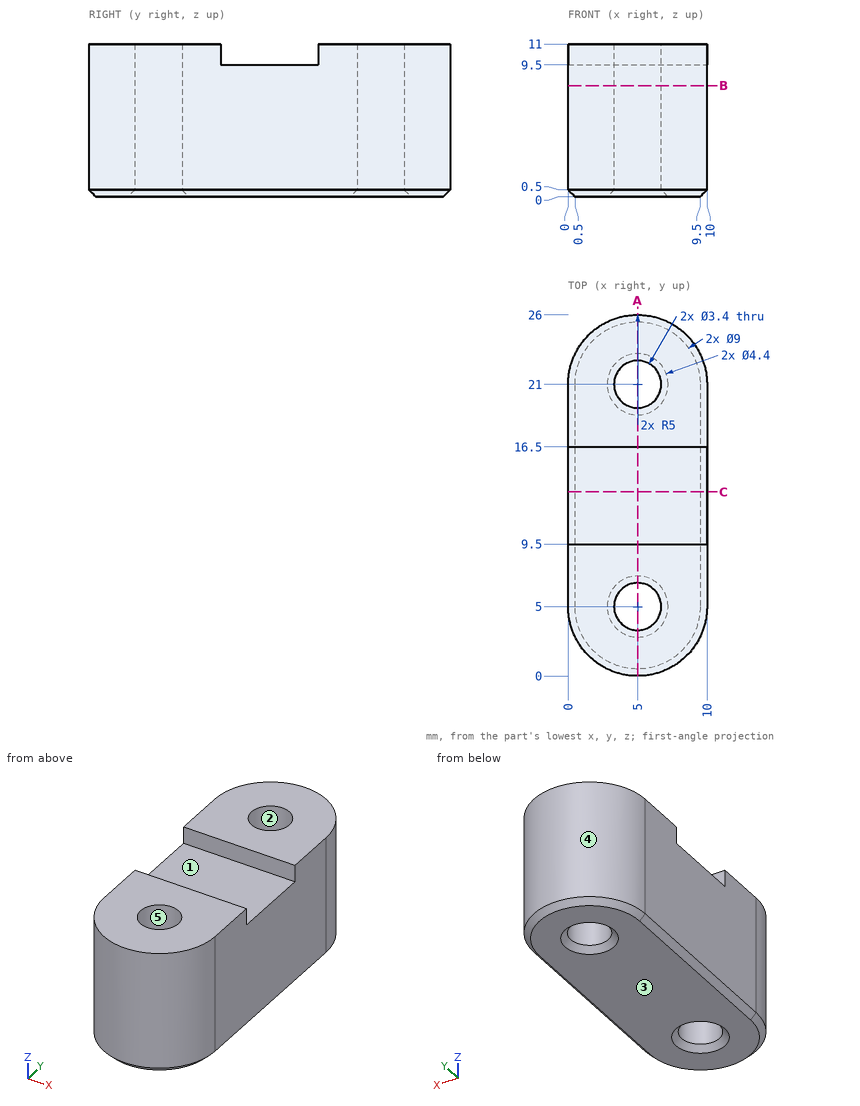
Geometry: see drawing. Coordinates: mm, zero at the bounding-box minimum. A direction names the side the tool comes from. Round coordinates to 2 decimals unless told otherwise and drop trailing zeros. Order: outer loops, then holes, each group sorted by start corner. A loop starts at its lowest first (then second) coordinate and runs counter-clockwise, first axis right, second up. Notation, with made-up numbers: (-15.5, 38) - (23.5, 38) arc R20 cw to (23.5, 56) - close; hole circle Ø10 at (26, 21). An arc over 180 degrees is marked (long way). Use a Markdown table: item, result. Add a question column.
1. First-contact query: pin 1 (0.8 mm diameter, centred on x = 3, z = 10, fed in from -Y); pin 2 (2 mm diameter, centred on x = 3.5, y = 12.5, fed in from +Z); pin 3 (2.5 mm diameter, centred on x = 5, y = 21, fed in from +Z). Flat tips, straight axial feed; report the tip coordinate or a pass-through.
2. Mould query, pull axis X, two halves, no side actions, for the marked faces 3, 4 and 5. Classes: +X half, -X half, draft (parallel to the pull), parting line (faces both ways), or undercut.
3. Section query A-A (x = 5). Return the cut outline in (y, z), then the cut area to 3 significant figures.
4. Set-up query: the marked faces 1 and 2. Return all of +Z, -Z, +X, -X, +Y, -Y with unobstructed straight access to the full face (end or side cutting, diameter ignored); none if empty.
5. Section query C-C (y = 13.25). Return the cut outline in (x, z), then the cut area to 4 significant figures.
6. Section query B-B (z = 8). Return the cut outline in (x, y).
7. Line query: probe 1 along Y at (x, z) = (5, 6.25); probe 2 along Z at (x, y) = (2.75, 12.25); probe 3 along Y at (x, z) = (7.75, 10.75). Output: solid intervals per line, ascending.
Derived:
| question | item | result |
|---|---|---|
| 1 | pin 1 | y = 0.26 |
| 1 | pin 2 | z = 9.5 |
| 1 | pin 3 | through |
| 2 | face 3 | draft |
| 2 | face 4 | parting line |
| 2 | face 5 | undercut |
| 3 | outline | (0, 0.5) - (0.5, 0) - (2.8, 0) - (3.3, 0.5) - (3.3, 11) - (0, 11) - close; (6.7, 0.5) - (7.2, 0) - (18.8, 0) - (19.3, 0.5) - (19.3, 11) - (16.5, 11) - (16.5, 9.5) - (9.5, 9.5) - (9.5, 11) - (6.7, 11) - close; (22.7, 0.5) - (23.2, 0) - (25.5, 0) - (26, 0.5) - (26, 11) - (22.7, 11) - close |
| 3 | area | 200 mm2 |
| 4 | face 1 | +Z, +X, -X |
| 4 | face 2 | +Z, -Z |
| 5 | outline | (0, 0.5) - (0.5, 0) - (9.5, 0) - (10, 0.5) - (10, 9.5) - (0, 9.5) - close |
| 5 | area | 94.75 mm2 |
| 6 | outline | (0, 5) arc R5 ccw to (10, 5) - (10, 21) arc R5 ccw to (0, 21) - close; hole circle Ø3.4 at (5, 5); hole circle Ø3.4 at (5, 21) |
| 7 | probe 1 | 0 to 3.3, 6.7 to 19.3, 22.7 to 26 |
| 7 | probe 2 | 0 to 9.5 |
| 7 | probe 3 | 0.82 to 9.5, 16.5 to 25.18 |
